Geometry: final body of the model. Coordinates: model frame, mm. A direction names the side the tool comes from. Coordinates: 2 decimals unless noted, no trailing zeros. Write each loop counter-clockwise with the first axis right and the second up, starting at its lowest first coordinate (ties: lowest second). Pieces come first, ordered by that corner, then holes. Notation, with made-up numbers: (52, 7) -> (89, 7) arc R18 ccw to (89, 31) -> close; hole circle Ø4 at (41.25, 36). An arc over 180 degrees is marked (long way). One line per item, written item: value.
```python
from build123d import *

# Parameters (mm, degrees)
SKETCH1_W           = 20.75
SKETCH1_H           = 48
SKETCH1_R           = 1.675
BOSS_EXTRUDE1_DEPTH = 6
SKETCH2_W           = 30
SKETCH2_H           = 48
BOSS_EXTRUDE2_DEPTH = 4
SKETCH3_R           = 8.25
CUT_EXTRUDE1_DEPTH  = 6
BOSS_EXTRUDE3_START = -26.5
BOSS_EXTRUDE3_DEPTH = 5
SKETCH5_R           = 2.925
CUT_EXTRUDE2_DEPTH  = 3
SKETCH6_W           = 4
SKETCH6_H           = 5
CUT_EXTRUDE3_DEPTH  = 34


with BuildPart() as part:
    # Sketch1 → Boss-Extrude1 (new body)
    with BuildSketch(Plane.XY):
        with Locations((10.375, 24)):
            Rectangle(SKETCH1_W, SKETCH1_H)
        with Locations((16.75, 34)):
            Circle(SKETCH1_R, mode=Mode.SUBTRACT)
        with Locations((16.75, 4)):
            Circle(SKETCH1_R, mode=Mode.SUBTRACT)
    extrude(amount=BOSS_EXTRUDE1_DEPTH)

    # Sketch2 → Boss-Extrude2 (add)
    with BuildSketch(Plane.ZY):
        with Locations((15, 24)):
            Rectangle(SKETCH2_W, SKETCH2_H)
    extrude(amount=-BOSS_EXTRUDE2_DEPTH)

    # Sketch3 → Cut-Extrude1 (cut)
    with BuildSketch(Plane.ZY):
        with Locations((18, 37)):
            Circle(SKETCH3_R)
        with Locations((18, 11)):
            Circle(SKETCH3_R)
    extrude(amount=-CUT_EXTRUDE1_DEPTH, mode=Mode.SUBTRACT)

    # Sketch4 → Boss-Extrude3 (add)
    with BuildSketch(Plane(origin=(0, 48, 0), x_dir=(1, 0, 0), z_dir=(0, 1, 0)).offset(BOSS_EXTRUDE3_START)):
        Polygon((4, -18), (4, -6), (18.555883802, -6), align=None)
    extrude(amount=BOSS_EXTRUDE3_DEPTH)

    # Sketch5 → Cut-Extrude2 (cut)
    with BuildSketch(Plane.XY.offset(6)):
        with Locations((16.75, 34)):
            Circle(SKETCH5_R)
        with Locations((16.75, 4)):
            Circle(SKETCH5_R)
    extrude(amount=-CUT_EXTRUDE2_DEPTH, mode=Mode.SUBTRACT)

    # Sketch6 → Cut-Extrude3 (cut)
    with BuildSketch(Plane(origin=(4, 0, 0), x_dir=(0, 0, -1), z_dir=(1, 0, 0))):
        with Locations((-16, 24)):
            Rectangle(SKETCH6_W, SKETCH6_H)
    extrude(amount=CUT_EXTRUDE3_DEPTH, mode=Mode.SUBTRACT)


solid = part.part
```
(1) Section B-B (z = 18). Return the cut outline in (x, y).
Responses:
outline: (0, 0) -> (4, 0) -> (4, 2.75) -> (0, 2.75) -> close; (0, 19.25) -> (4, 19.25) -> (4, 28.75) -> (0, 28.75) -> close; (0, 45.25) -> (4, 45.25) -> (4, 48) -> (0, 48) -> close
(2) Reachability of faces 1 (the flat face through (12, 30, 6)), 2 (the flat face through (10, 26.5, 9)), 3 (the flat face through (6, 24, 14)), 4 (the cylindrical face through (19.54, 34.88, 4.52)), 5 (the flat face through (10, 21.5, 9)) from +Z, -Z, +X, -X, +Y, -Y: full face, straight path, thin tool, end or side. Return the list, or none.
Responses:
face 1: +Z, +X
face 2: +Z, +X, +Y
face 3: +Z, +X, +Y, -Y
face 4: +Z
face 5: +Z, +X, -Y
(3) Pull-direction query (X, two-part tool) for faces 6 (the flat face through (3, 0, 8)), 7 (the flat face through (13.772, 23.965, 9.944)), 8 (the cylindrical face through (18.3, 3.36, 1.48)); classes: released by +X, released by -X, zero draft, split by the parting line, or undercut.
Responses:
face 6: zero draft
face 7: released by +X
face 8: undercut
(4) Line query: line 1 (Y direction, x = 16.75, z = 2.25) (3 decimals); line 2 (Y direction, x = 16.75, z = 4.95) (3 decimals); line 3 (X direction, y = 34, z = 1.45) (3 decimals). Output: solid intervals per line, ascending. Write a range as [from, to].
Responses:
line 1: y = [0, 2.325], [5.675, 32.325], [35.675, 48]
line 2: y = [0, 1.075], [6.925, 31.075], [36.925, 48]
line 3: x = [0, 15.075], [18.425, 20.75]
(5) Section C-C (x = 16.75). Return the cut outline in (y, z) (3 decimals).
Responses:
outline: (0, 0) -> (2.325, 0) -> (2.325, 3) -> (1.075, 3) -> (1.075, 6) -> (0, 6) -> close; (5.675, 0) -> (32.325, 0) -> (32.325, 3) -> (31.075, 3) -> (31.075, 6) -> (26.5, 6) -> (26.5, 7.489) -> (21.5, 7.489) -> (21.5, 6) -> (6.925, 6) -> (6.925, 3) -> (5.675, 3) -> close; (35.675, 0) -> (48, 0) -> (48, 6) -> (36.925, 6) -> (36.925, 3) -> (35.675, 3) -> close
(6) First-contact query: pin 1 (3 mm diameter, centred on x = 16.75, y = 4, fed in from +Z); pin 2 (2.5 mm diameter, centred on x = 6.5, y = 24.5, fed in from +Z); pin 3 (1.5 mm diameter, centred on x = 16, z = 8, fed in from -Y); pin 4 (5 mm diameter, centred on x = 13.5, y = 15, fed in from +Z). Flat tips, straight axial feed; report the tip coordinate or a pass-through.
Responses:
pin 1: passes through
pin 2: stops at z = 14
pin 3: stops at y = 21.5
pin 4: stops at z = 6
(7) Section A-A (y = 11). Return the cut outline in (x, z).
Responses:
outline: (0, 0) -> (20.75, 0) -> (20.75, 6) -> (4, 6) -> (4, 9.75) -> (0, 9.75) -> close; (0, 26.25) -> (4, 26.25) -> (4, 30) -> (0, 30) -> close
(8) Section D-D (x = 2). Return the cut outline in (y, z).
Responses:
outline: (0, 0) -> (48, 0) -> (48, 30) -> (0, 30) -> close; hole circle Ø16.5 at (11, 18); hole circle Ø16.5 at (37, 18)
